Study the drawing (mm; zero at the part's minimum x, y, z) and answer. A direction names the side the tool comes from. Coordinates: 2 decimals unless noted, no trailing zeros. Write each loop counter-clockwise with the first axis right and the second up, starting at its lowest first coordinate (ties: lowest second). Pieces come first, ordered by that corner, then holes. Notation, with made-up numbers: (50.25, -36.75) -> (78.25, -36.75) arc R16 ccw to (78.25, -24.75) -> close; hole circle Ø5 at (52, -22). An arc over 180 degrees is marked (long way). Write each question's results on one line, items separated by ' | '. Start each with the question number.
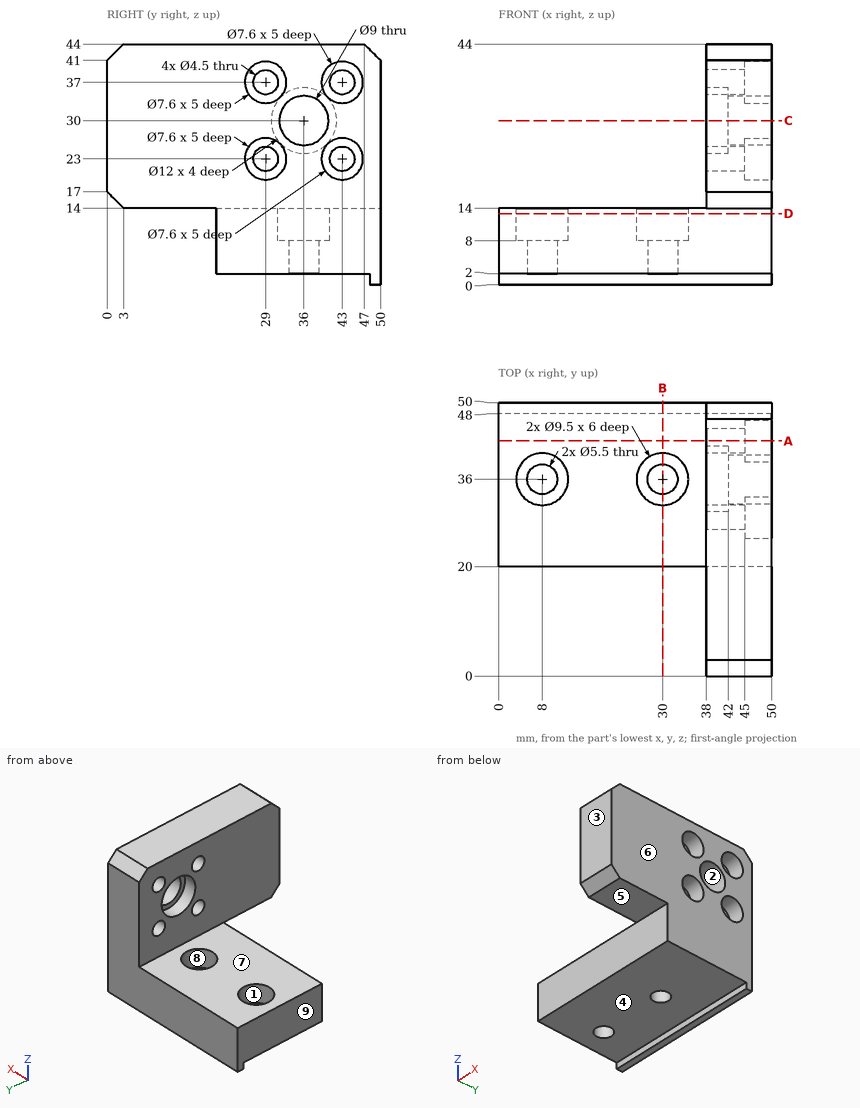
1. Determine the mould class of the marked faces 1, 2, 3 and 4 for opening direction Y: pulls with the +Y half, pulls with the -Y half, needs draft (parallel to the pull), parting line crosses it, or undercut.
2. Find section D-D on z = 13. Give the vertices of the cut face in (x, y), and give its area (3 significant figures).
3. Given pin 1 Ø13 at (y, z) = (35, 28.5) entering from -X; pin 2 Ø1.6 at (x, z) = (33.5, 0.5) entering from -Y; pin 3 Ø3 at (x, y) = (9.5, 36.5) entering from +Z; pin 4 Ø3.5 at (y, z) = (43, 37) entering from -X, each flat-ended and moving along its own axis, determine where each tip first touches the part or whether it passes through.
4. Find section C-C on z = 30. Give the vertices of the cut face in (x, y), and give its area (3 significant figures).
5. For the marked faces 5, 6, 7, 8 and 9, determine the directions among +Z, -Z, +X, -X, +Y, -Y from which every point of the face is accessible in a straight line to the end or side of a thin tool.
6. Find section A-A on y = 43. Give the vertices of the cut face in (x, z).
7. Find the intervals of material crossed by L1, parallel to Y at x = 48.8, z = 23; L2, parallel to Y at x = 42, z = 37; L3, parallel to Y at x = 45, z = 30, in increasing order.
8. Find section B-B on x = 30. Give the vertices of the cut face in (y, z), and give its area (3 significant figures).
Ans:
1) face 1: undercut | face 2: undercut | face 3: pulls with the -Y half | face 4: needs draft
2) outline: (0, 20) -> (50, 20) -> (50, 50) -> (0, 50) -> close; hole circle Ø9.5 at (8, 36); hole circle Ø9.5 at (30, 36) | area: 1,360 mm²
3) pin 1: stops at x = 38 | pin 2: stops at y = 48 | pin 3: stops at z = 8 | pin 4: passes through
4) outline: (38, 0) -> (50, 0) -> (50, 31.5) -> (42, 31.5) -> (42, 30) -> (38, 30) -> close; (38, 42) -> (42, 42) -> (42, 40.5) -> (50, 40.5) -> (50, 50) -> (38, 50) -> close | area: 480 mm²
5) face 5: -Z, +X, -X, -Y | face 6: +Z, -Z, +X, +Y, -Y | face 7: +Z, -X, +Y, -Y | face 8: +Z | face 9: +Z, -Z, -X, +Y, -Y
6) outline: (0, 2) -> (50, 2) -> (50, 19.2) -> (45, 19.2) -> (45, 20.75) -> (38, 20.75) -> (38, 14) -> (0, 14) -> close; (38, 25.25) -> (45, 25.25) -> (45, 26.8) -> (50, 26.8) -> (50, 33.2) -> (45, 33.2) -> (45, 34.75) -> (38, 34.75) -> close; (38, 39.25) -> (45, 39.25) -> (45, 40.8) -> (50, 40.8) -> (50, 44) -> (38, 44) -> close
7) L1: y = 0 to 25.2, 32.8 to 39.2, 46.8 to 50 | L2: y = 0 to 26.75, 31.25 to 40.75, 45.25 to 50 | L3: y = 0 to 31.5, 40.5 to 50
8) outline: (20, 2) -> (33.25, 2) -> (33.25, 8) -> (31.25, 8) -> (31.25, 14) -> (20, 14) -> close; (38.75, 2) -> (48, 2) -> (48, 0) -> (50, 0) -> (50, 14) -> (40.75, 14) -> (40.75, 8) -> (38.75, 8) -> close | area: 274 mm²
